Read the model definition and answer for the solid it produces. Units are mm, in the model's axes. Coordinates: 2 decimals unless noted, no trailing zeros. Write each loop counter-clockwise with the first axis right and the second up, starting at its lowest first coordinate (ties: lowest second). Pieces come first, ordered by that corner, then holes.
(1) Find the intervals of material crossed by probe 1 along Z at (x, y) = (-173, 27.5); probe 2 along Z at (x, y) = (-206.5, 36); probe 3 along X at (y, z) = (24.5, -291.5), in increasing order.
(2) Section A-A on y = 41 is taken. Write down the section's boundary in (x, z).
(3) The mould has two halves that part along Z. Classify faces 1 (the cylindrical face through (-163.161, 9.021, -8.555)), 2 (the cylindrical face through (-9.6, 80.4, -322.1)), 3 (the flat face through (-137, 159.4, -137)): +Z half, -Z half, draft (parallel to the pull), parting line (faces both ways), or undercut.
(4) Given pin 1 (1.5 mm diameter, centred on x = -279.5, z = -157.5, fed in from -Y); pin 2 (5 mm diameter, centred on x = -291.5, z = -155, fed in from +Y); pin 3 (6 mm diameter, centred on y = 141, z = -246, fed in from +X), each flat-ended and moving along its own axis, determine where each tip first touches the part or whether it passes through.
from build123d import *

# Parameters (mm, degrees)
BOSS_EXTRUDE1_DEPTH = 159.4
FILLET1_R           = 30


with BuildPart() as part:
    # Sketch1 → Boss-Extrude1 (new body)
    with BuildSketch(Plane(origin=(0, 0, 0), x_dir=(1, 0, 0), z_dir=(0, 1, 0))):
        with BuildLine():
            Line((-331.6, 0), (0, 0))
            Line((0, 0), (0, 331.6))
            ThreePointArc((0, 331.6), (-234.476608641, 234.476608641), (-331.6, 0))
        make_face()
    extrude(amount=BOSS_EXTRUDE1_DEPTH)

    # Fillet1
    fillet1_edges = [part.edges().sort_by_distance(p)[0] for p in [
        (-165.8, 159.4, 0),
        (-165.8, 0, 0),
        (-234.476608641, 0, -234.476608641),
        (0, 0, -165.8),
        (0, 159.4, -165.8),
        (0, 79.7, 0),
        (-331.6, 79.7, 0),
        (0, 79.7, -331.6),
        (-234.476608641, 159.4, -234.476608641),
    ]]
    fillet(fillet1_edges, radius=FILLET1_R)


solid = part.part
Response:
1. probe 1: z = -282.77 to -0.1
1. probe 2: z = -259.45 to 0
1. probe 3: x = -157 to -0.51
2. outline: (-329.96, -32.98) arc R331.6 ccw to (-32.98, -329.96) arc R30 ccw to (0, -300.1) - (0, -30) arc R30 ccw to (-30, 0) - (-300.1, 0) arc R30 ccw to start
3. face 1: +Z half
3. face 2: -Z half
3. face 3: draft
4. pin 1: stops at y = 6.36
4. pin 2: stops at y = 144.28
4. pin 3: stops at x = -1.26
